Drawing for the job (mm, zero at the part's lowest x, y, z). A direction names the side the tool comes from. Round coordinates to 2 decimals unless told otherwise and drop trailing zeros. Loops run counter-clockwise (first coordinate to the right, second up) from the corner with the lowest first, then second, coordinate; pieces in that order, holes last. Notation, with made-up numbers: (-31, 8) -> (-5, 8) arc R16 ccw to (-5, 38) -> close; hole circle Ø6 at (-21.75, 31.25). An arc over 180 degrees is marked (long way). Put each result on its own line as item: value. Start each with the question number.
Item 1: Cut at D-D, the plane z = 20.25. List the corners of the cut face in (x, y).
Item 2: Drill centre lines: probe 1 along Z at (x, y) = (4.5, 4); probe 2 along Z at (x, y) = (5.3, 2.8); probe 3 along X at (y, z) = (0.65, 9.25). Where is each one in solid material? Low to high. Write a range as [from, to].
Item 3: Cut at A-A, the plane x = 3. List the corners of the cut face in (y, z).
Item 4: Flat gauge pins, fed straight in: pin 1 Ø3 at (x, z) = (3.5, 3.5) entering from -Y; pin 2 Ø1.5 at (x, z) = (1, 4.5) entering from +Y. Where does each tip first touch, or does it go through?
Item 5: Cut at C-C, the plane z = 6.25. List the corners of the cut face in (x, y).
Item 6: Tool access for the marked faces 1, 2 and 3: list every direction of +Z, -Z, +X, -X, +Y, -Y with a clear straight run to the whole face (end or side of a thin tool).
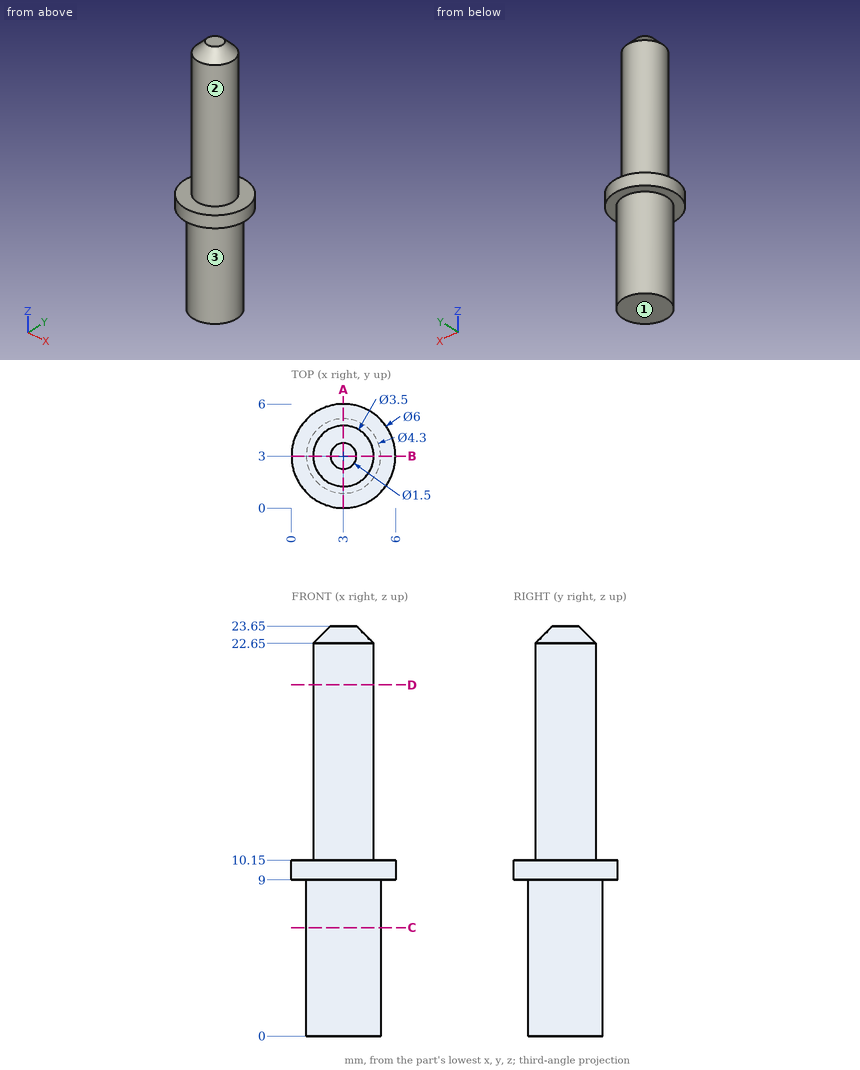
Reply:
1. outline: circle Ø3.5 at (3, 3)
2. probe 1: z = [0, 10.15]
2. probe 2: z = [9, 10.15]
2. probe 3: x = [1.14, 4.86]
3. outline: (0, 9) -> (0.85, 9) -> (0.85, 0) -> (5.15, 0) -> (5.15, 9) -> (6, 9) -> (6, 10.15) -> (4.75, 10.15) -> (4.75, 22.65) -> (3.75, 23.65) -> (2.25, 23.65) -> (1.25, 22.65) -> (1.25, 10.15) -> (0, 10.15) -> close
4. pin 1: stops at y = 0.85
4. pin 2: stops at y = 4.75
5. outline: circle Ø4.3 at (3, 3)
6. face 1: -Z, +X, -X, +Y, -Y
6. face 2: +Z
6. face 3: -Z
